Geometry: final body of the model. Coordinates: model frame, mm. A direction names the side the tool comes from. Round coordinates to 2 decimals unless told otherwise and drop trailing zeros. Loops run counter-clockwise (first coordinate to the right, second up) from the corner with the lowest first, then second, coordinate; pieces in that order, holes last. Notation, with made-up numbers: (-13.75, -7) - (12.25, -7) arc R20 ccw to (12.25, 14) - close; hole circle Ø9 at (30, 50). An arc over 180 degrees is marked (long way). Write item = value, one per line. Start each with the question number.
Item 1: Access query for faces 1 (the flat face through (26, -3.9, -20)), 2 (the flat face through (27.1, 0, 0)), 3 (the flat face through (20.4, 20.3, -20.5)), 4 (the flat face through (26, 3.9, -2)), 5 (the flat face through (7, 23.1, -12)). Directions: +Z, -Z, +X, -X, +Y, -Y. A direction counts if a zero-diameter tool reaches every point of the face in a straight line with its end or side. Return the directions, or none.
Item 2: Line query: line 1 (X direction, y = -8, z = -14); line 2 (X direction, y = 3, z = -15); line 3 (Z direction, x = 14.5, y = -10). Output: solid intervals per line, ascending. Write a range as from..to.
Item 3: Section A-A (z = -17). Return loops of the section in (x, y), plus the area to 3 significant figures.
Item 4: First-contact query: pin 1 (1.6 mm diameter, centred on x = 26, z = -36.5, fed in from -Y); pin 2 (6 mm diameter, centred on y = -5.5, z = -15.5, fed in from -X); pin 3 (6 mm diameter, centred on x = -1.5, z = -10, fed in from -Y). Flat tips, straight axial feed; report the tip coordinate or a pass-through.
from build123d import *

# Parameters (mm, degrees)
F0_W      = 42.2
F0_H      = 42.2
F1_DEPTH  = 5
F2_DEPTH  = 40
F3_DEPTH  = 2
F5_DEPTH  = 25
F4_W      = 3.9
F4_H      = 6.5
F6_DEPTH  = 2
F7_SIZE   = 0.5
F8_SIZE   = 35
F9_DEPTH  = 16.75
F10_DEPTH = 21.75
F11_DEPTH = 25
F12_SIZE  = 1.5


# Not quite as in the source:
# - a feature names something its author has since deleted; it is built from what else it names


with BuildPart() as f1:
    # F0 (on Top) → F1 (new body)
    with BuildSketch(Plane.XY):
        Rectangle(F0_W, F0_H)
        with BuildLine():
            ThreePointArc((-15.5, 13.75), (-16.7374368671, 16.7374368671), (-13.75, 15.5))
            Line((-13.75, 15.5), (0, 15.5))
            Line((0, 15.5), (13.75, 15.5))
            ThreePointArc((13.75, 15.5), (15.5, 17.25), (17.25, 15.5))
            ThreePointArc((17.25, 15.5), (16.7374368671, 14.2625631329), (15.5, 13.75))
            Line((15.5, 13.75), (15.5, 0))
            Line((15.5, 0), (15.5, -13.75))
            ThreePointArc((15.5, -13.75), (16.7374368671, -14.2625631329), (17.25, -15.5))
            ThreePointArc((17.25, -15.5), (15.5, -17.25), (13.75, -15.5))
            Line((13.75, -15.5), (0, -15.5))
            Line((0, -15.5), (-13.75, -15.5))
            ThreePointArc((-13.75, -15.5), (-16.7374368671, -16.7374368671), (-15.5, -13.75))
            Line((-15.5, -13.75), (-15.5, 0))
            Line((-15.5, 0), (-15.5, 13.75))
        make_face(mode=Mode.SUBTRACT)
        Polygon((-21.1, 21.1), (21.1, 21.1), (21.1, -21.1), (23.1, -21.1), (23.1, 23.1), (-21.1, 23.1), align=None)
        with BuildLine():
            Line((0, 15.5), (-13.75, 15.5))
            ThreePointArc((-13.75, 15.5), (-14.2625631329, 14.2625631329), (-15.5, 13.75))
            Line((-15.5, 13.75), (-15.5, 0))
            ThreePointArc((-15.5, 0), (-10.9601551084, 10.9601551084), (0, 15.5))
        make_face()
        with BuildLine():
            ThreePointArc((0, -15.5), (-10.9601551084, -10.9601551084), (-15.5, 0))
            Line((-15.5, 0), (-15.5, -13.75))
            ThreePointArc((-15.5, -13.75), (-14.2625631329, -14.2625631329), (-13.75, -15.5))
            Line((-13.75, -15.5), (0, -15.5))
        make_face()
        with BuildLine():
            Line((15.5, -13.75), (15.5, 0))
            ThreePointArc((15.5, 0), (10.9601551084, -10.9601551084), (0, -15.5))
            Line((0, -15.5), (13.75, -15.5))
            ThreePointArc((13.75, -15.5), (14.2625631329, -14.2625631329), (15.5, -13.75))
        make_face()
        with BuildLine():
            Line((13.75, 15.5), (0, 15.5))
            ThreePointArc((0, 15.5), (10.9601551084, 10.9601551084), (15.5, 0))
            Line((15.5, 0), (15.5, 13.75))
            ThreePointArc((15.5, 13.75), (14.2625631329, 14.2625631329), (13.75, 15.5))
        make_face()
    extrude(amount=F1_DEPTH)

    # F0 (on Top) → F2 (join)
    with BuildSketch(Plane.XY):
        Polygon((-21.1, 21.1), (21.1, 21.1), (21.1, -21.1), (23.1, -21.1), (23.1, 23.1), (-21.1, 23.1), align=None)
    extrude(amount=-F2_DEPTH)

    # F3 (add): a face of the model
    f3_faces = [f1.faces().sort_by_distance(p)[0] for p in [
        (23.1, 1, -17.5),
    ]]
    extrude(f3_faces, amount=F3_DEPTH)

    # F4 (on face) → F5 (cut)
    with BuildSketch(Plane.YZ.offset(25.1)):
        with BuildLine():
            ThreePointArc((4.25, -10), (3.00520382, -6.99479618), (0, -5.75))
            Line((0, -5.75), (0, -10))
            Line((0, -10), (0, -14.25))
            ThreePointArc((0, -14.25), (3.00520382, -13.00520382), (4.25, -10))
        make_face()
        with BuildLine():
            Line((0, -10), (0, -5.75))
            ThreePointArc((0, -5.75), (-4.25, -10), (0, -14.25))
            Line((0, -14.25), (0, -10))
        make_face()
        with BuildLine():
            Line((0, -30), (0, -34.25))
            ThreePointArc((0, -34.25), (3.00520382, -33.00520382), (4.25, -30))
            Line((4.25, -30), (0, -30))
        make_face()
        with BuildLine():
            ThreePointArc((0, -25.75), (-4.25, -30), (0, -34.25))
            Line((0, -34.25), (0, -30))
            Line((0, -30), (0, -25.75))
        make_face()
        with BuildLine():
            ThreePointArc((4.25, -30), (3.00520382, -26.99479618), (0, -25.75))
            Line((0, -25.75), (0, -30))
            Line((0, -30), (4.25, -30))
        make_face()
    extrude(amount=-F5_DEPTH, mode=Mode.SUBTRACT)

    # F4 (on face) → F6 (join)
    with BuildSketch(Plane.YZ.offset(25.1)):
        with Locations((1.95, -20)):
            Rectangle(F4_W, F4_H)
        with Locations((-1.95, -20)):
            Rectangle(F4_W, F4_H)
    extrude(amount=F6_DEPTH)

    # F7
    f7_edges = [f1.edges().sort_by_distance(p)[0] for p in [
        (21.1, -4.25, -30),
        (21.1, -4.25, -10),
        (0, -15.5, 5),
        (0, -15.5, 0),
        (-17.25, 15.5, 0),
        (-15.5, -17.25, 0),
        (17.25, -15.5, 0),
        (15.5, 17.25, 0),
    ]]
    chamfer(f7_edges, length=F7_SIZE)

    # F8
    f8_edges = [f1.edges().sort_by_distance(p)[0] for p in [
        (-21.1, 22.1, -40),
    ]]
    chamfer(f8_edges, length=F8_SIZE)

    # F9 (add): a face of the model
    f9_faces = [f1.faces().sort_by_distance(p)[0] for p in [
        (26.1, 0, -23.25),
    ]]
    extrude(f9_faces, amount=F9_DEPTH)

    # F10 (add): a face of the model
    f10_faces = [f1.faces().sort_by_distance(p)[0] for p in [
        (26.1, 0, -16.75),
    ]]
    extrude(f10_faces, amount=F10_DEPTH)

    # F11 (cut): faces of the model
    f11_faces = [f1.faces().sort_by_distance(p)[0] for p in [
        (25.1, 0, -10),
        (25.1, 0, -30),
    ]]
    extrude(f11_faces, amount=-F11_DEPTH, mode=Mode.SUBTRACT)

    # F12
    f12_edges = [f1.edges().sort_by_distance(p)[0] for p in [
        (21.1, 0, 0),
        (21.1, 21.1, -20),
        (0, 21.1, 0),
    ]]
    chamfer(f12_edges, length=F12_SIZE)


solid = f1.part
Taken from the geometry:
q1.face_1 = +Z, -Z, +X, -Y
q1.face_2 = +Z, -Z, +X, +Y, -Y
q1.face_3 = -Z, -X, -Y
q1.face_4 = +Z, -Z, +X, +Y
q1.face_5 = +Z, -Z, +X, -X, +Y
q2.line_1 = 21.1..25.1
q2.line_2 = 21.1..27.1
q2.line_3 = 0..5
q3.outline = (-9.1, 21.1) - (19.6, 21.1) - (21.1, 19.6) - (21.1, -21.1) - (25.1, -21.1) - (25.1, -3.9) - (27.1, -3.9) - (27.1, 3.9) - (25.1, 3.9) - (25.1, 23.1) - (-9.1, 23.1) - close
q3.area = 254 mm^2
q4.pin_1 = -3.9
q4.pin_2 = 21.1
q4.pin_3 = 21.1
